Work out the finished part from the listing and answer in its coordinate system (mm). Coordinates: 2 decimals unless noted, no trailing zeros. Write each loop counter-clockwise with the first axis right and the second up, starting at its lowest first coordinate (ties: lowest second). Pieces come first, ordered by that corner, then holes. Notation, with made-up numbers: (44, 36) - (76, 36) arc R12 cw to (76, 53) - close; hole circle Ø6 at (86, 40.25). An arc over 180 degrees is marked (long way). Answer as a JSON object with one key per item and string values. Group by question number.
from build123d import *

# Parameters (mm, degrees)
SKETCH1_R           = 3.850000047
BOSS_EXTRUDE1_DEPTH = 44.45
SKETCH4_R           = 0.45
CUT_EXTRUDE1_DEPTH  = 10.16
LPATTERN1_COUNT     = 7
LPATTERN1_PITCH     = 5


with BuildPart() as part:
    # Sketch1 → Boss-Extrude1 (new body)
    with BuildSketch(Plane(origin=(0, 0, 0), x_dir=(1, 0, 0), z_dir=(0, 1, 0))):
        Circle(SKETCH1_R)
    extrude(amount=BOSS_EXTRUDE1_DEPTH)

    # Sketch4 → Cut-Extrude1 (cut)
    with BuildSketch(Plane.XY.offset(5.08)):
        with Locations((0, 8.566631878)):
            Circle(SKETCH4_R)
    cut_extrude1 = extrude(amount=-CUT_EXTRUDE1_DEPTH, mode=Mode.SUBTRACT)

    # LPattern1: Cut-Extrude1 ×7
    with Locations(*[(0, i * LPATTERN1_PITCH, 0) for i in range(1, LPATTERN1_COUNT)]):
        add(cut_extrude1, mode=Mode.SUBTRACT)


solid = part.part
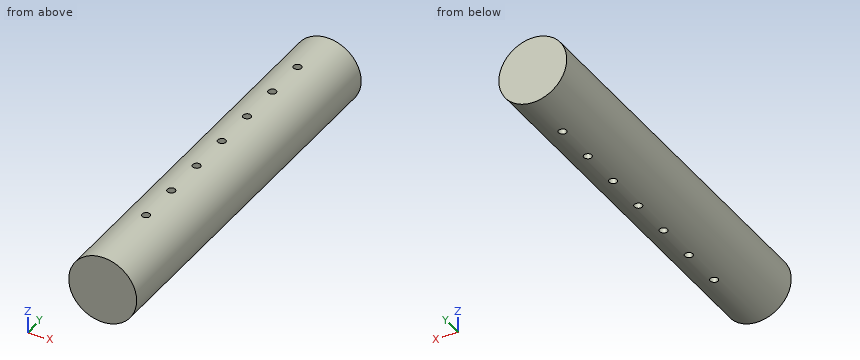
Q1. Section A-A on x = 0 is taken. Count the separate pieces of the cut face and the enclosed holes in it, plus the area to 3 significant figures.
Q2. Consider L1, parallel to Z at x = -0.25, y = 16.5; L2, parallel to Z at x = -2.5, y = 30.5; L3, parallel to X at y = 29.5, z = -1.5. Determine where each line is inside the solid, lowest interval first. Write a range as from..to.
Q3. Section D-D on z = -1 is taken. Determine the outline of the cut face in (x, y).
Q4. Section C-C on y = 32 is taken. Determine the outline of the cut face in (x, z).
Q5. Flat-ended cylindrical pins translate along their axes: pin 1 Ø1 at (y, z) = (11, -1) entering from -X; pin 2 Ø1 at (y, z) = (19.5, -2.5) entering from +X. Find the tip coordinate at first contact, or state that the pin passes through.
Q6. Section B-B on z = 2.25 is taken. Determine the outline of the cut face in (x, y).
Numbers:
{
 "1": {"separate pieces": "8", "enclosed holes": "0", "area": "294 mm²"},
 "2": {"L1": "z = -3.84..3.84", "L2": "z = -2.93..2.93", "L3": "x = -3.55..3.55"},
 "3": {"outline": "(-3.72, 0) - (3.72, 0) - (3.72, 44.45) - (-3.72, 44.45) - close; hole circle Ø0.9 at (0, 8.57); hole circle Ø0.9 at (0, 13.57); hole circle Ø0.9 at (0, 18.57); hole circle Ø0.9 at (0, 23.57); hole circle Ø0.9 at (0, 28.57); hole circle Ø0.9 at (0, 33.57); hole circle Ø0.9 at (0, 38.57)"},
 "4": {"outline": "circle Ø7.7 at (0, 0)"},
 "5": {"pin 1": "stops at x = -3.82", "pin 2": "stops at x = 3.29"},
 "6": {"outline": "(-3.12, 0) - (3.12, 0) - (3.12, 44.45) - (-3.12, 44.45) - close; hole circle Ø0.9 at (0, 8.57); hole circle Ø0.9 at (0, 13.57); hole circle Ø0.9 at (0, 18.57); hole circle Ø0.9 at (0, 23.57); hole circle Ø0.9 at (0, 28.57); hole circle Ø0.9 at (0, 33.57); hole circle Ø0.9 at (0, 38.57)"}
}
